Read the model definition and answer for the solid it produces. Units are mm, in the model's axes. A direction names the side the tool comes from. Round coordinates to 2 decimals unless told otherwise and drop trailing zeros. Order: outer loops, then holes, each group sorted by start corner. A loop starts at its lowest first (then second) coordinate and runs counter-clockwise, first axis right, second up. Notation, with made-up numbers: (22, 19.5) - (40, 19.5) arc R21 cw to (40, 25.5) - close; hole circle Ø5 at (47.25, -19.5). An arc over 180 degrees is marked (long way). One line per question, with ' | ' between items. Start each with the question number.
1) The part is cut by section B-B, the plane y = -30. Give the vertices of the cut face in (x, z).
2) The part is cut by section A-A, the plane x = 0. Give the vertices of the cut face in (y, z).
3) Straight lines are drawn through the part: line 1 (X direction, y = -8.7, z = 6); line 2 (X direction, y = -11.5, z = 6); line 3 (X direction, y = -13, z = 8.5). For each, find the intervals that lie inside material, in ascending order. Write a range as from..to.
4) The part is cut by section D-D, the plane x = 18. Give the vertices of the cut face in (y, z).
5) The part is cut by section C-C, the plane z = 6. Give the vertices of the cut face in (x, y).
6) The mould has two halves that part along Y. Classify faces 1 (the cylindrical face through (-51.29, -43.49, 6.08)), 2 (the flat face through (-31.4, 9.9, 12)), 3 (the cylindrical face through (-44.241, 25.877, 5.916)): pulls with the +Y half, pulls with the -Y half, needs draft (parallel to the pull), parting line crosses it, or undercut.
7) For faces 4 (the cylindrical face through (-37.69, 6.837, 5.916)), 5 (the flat face through (-52, -39, 6)), determine the directions among +Z, -Z, +X, -X, +Y, -Y from which every point of the face is accessible in a straight line to the end or side of a thin tool.
8) Flat-ended cylindrical pins translate along their axes: pin 1 (3.5 mm diameter, centred on x = -35.29, z = 6, fed in from -Y); pin 2 (2 mm diameter, centred on x = -14.5, z = 10, fed in from -Y); pin 3 (5 mm diameter, centred on x = -35.29, z = 6, fed in from +Y); pin 4 (4 mm diameter, centred on y = 22, z = 8.5, fed in from +X). Find the tip coordinate at first contact, or state that the pin passes through.
from build123d import *

# Parameters (mm, degrees)
F1_DEPTH = 12
F3_R     = 4
F3_R_2   = 2
F6_DEPTH = 100
F7_R     = 1


with BuildPart() as f1:
    # F0 (on Top) → F1 (new body)
    with BuildSketch(Plane.XY):
        with BuildLine():
            ThreePointArc((-30.9533166858, 9.9066738185), (32.5, 0), (-30.9533166858, -9.9066738185))
            ThreePointArc((-30.9533166858, -9.9066738185), (-36.1521865846, -6.4498953062), (-40.6700074334, -10.7588233268))
            ThreePointArc((-40.6700074334, -10.7588233268), (-44.1719937167, -25.6732051584), (-50.4508620887, -39.647413734))
            Line((-50.4508620887, -39.647413734), (-52, -35))
            Line((-52, -35), (-52, -45.9262987944))
            ThreePointArc((-52, -45.9262987944), (-43.3754164337, -29.3581013392), (-38.7212103105, -11.2686852631))
            ThreePointArc((-38.7212103105, -11.2686852631), (-38.6982701791, -11.0262325635), (-38.6558059993, -10.7864277375))
            ThreePointArc((-38.6558059993, -10.7864277375), (-35.9754973818, -8.4318261948), (-32.9297903997, -10.2897475302))
            ThreePointArc((-32.9297903997, -10.2897475302), (-32.8484099779, -10.5132023948), (-32.7849231086, -10.7423841283))
            ThreePointArc((-32.7849231086, -10.7423841283), (34.5, 0), (-32.7849231086, 10.7423841283))
            ThreePointArc((-32.7849231086, 10.7423841283), (-32.8484099779, 10.5132023948), (-32.9297903997, 10.2897475302))
            ThreePointArc((-32.9297903997, 10.2897475302), (-35.9754973818, 8.4318261948), (-38.6558059993, 10.7864277375))
            ThreePointArc((-38.6558059993, 10.7864277375), (-38.6982701791, 11.0262325635), (-38.7212103105, 11.2686852631))
            ThreePointArc((-38.7212103105, 11.2686852631), (-43.3754164337, 29.3581013392), (-52, 45.9262987944))
            Line((-52, 45.9262987944), (-52, 35))
            Line((-52, 35), (-50.4508620887, 39.647413734))
            ThreePointArc((-50.4508620887, 39.647413734), (-44.1719937167, 25.6732051584), (-40.6700074334, 10.7588233268))
            ThreePointArc((-40.6700074334, 10.7588233268), (-36.1521865846, 6.4498953062), (-30.9533166858, 9.9066738185))
        make_face()
        with BuildLine():
            ThreePointArc((-38.6558059993, -10.7864277375), (-38.6982701791, -11.0262325635), (-38.7212103105, -11.2686852631))
            ThreePointArc((-38.7212103105, -11.2686852631), (-38.6881506227, -11.0276049892), (-38.6558059993, -10.7864277375))
        make_face()
        with BuildLine():
            ThreePointArc((-38.6558059993, 10.7864277375), (-38.6881506227, 11.0276049892), (-38.7212103105, 11.2686852631))
            ThreePointArc((-38.7212103105, 11.2686852631), (-38.6982701791, 11.0262325635), (-38.6558059993, 10.7864277375))
        make_face()
        with BuildLine():
            ThreePointArc((-32.7849231086, -10.7423841283), (-32.8484099779, -10.5132023948), (-32.9297903997, -10.2897475302))
            ThreePointArc((-32.9297903997, -10.2897475302), (-32.8581361742, -10.5163152843), (-32.7849231086, -10.7423841283))
        make_face()
        with BuildLine():
            ThreePointArc((-32.7849231086, 10.7423841283), (-32.8581361742, 10.5163152843), (-32.9297903997, 10.2897475302))
            ThreePointArc((-32.9297903997, 10.2897475302), (-32.8484099779, 10.5132023948), (-32.7849231086, 10.7423841283))
        make_face()
    extrude(amount=F1_DEPTH)

    # F3 (on offset) → F4 (join, up to the next surface of F1)
    with BuildSketch(Plane.XZ.offset(15)):
        with Locations((-35.2927981995, 6)):
            Circle(F3_R)
        with Locations((-35.2927981995, 6)):
            Circle(F3_R_2, mode=Mode.SUBTRACT)
    extrude(until=Until.NEXT, dir=(0, 1, 0))

    # F5: F1 across plane


with BuildPart() as f1_1:
    add(f1.part)
    add(f1.part.mirror(Plane.XZ))

    # F3 (on offset) → F6 (cut)
    with BuildSketch(Plane.XZ.offset(15)):
        with Locations((-35.2927981995, 6)):
            Circle(F3_R_2)
    extrude(amount=-F6_DEPTH, mode=Mode.SUBTRACT)

    # F7
    f7_edges = [f1_1.edges().sort_by_distance(p)[0] for p in [
        (-52, -45.926299, 6),
        (-52, 45.926299, 6),
    ]]
    fillet(f7_edges, radius=F7_R)


solid = f1_1.part
Values:
1) outline: (-45.78, 0) - (-43.62, 0) - (-43.62, 12) - (-45.78, 12) - close; (-17.04, 0) - (-12.5, 0) - (-12.5, 12) - (-17.04, 12) - close; (12.5, 0) - (17.04, 0) - (17.04, 12) - (12.5, 12) - close
2) outline: (-34.5, 0) - (-32.5, 0) - (-32.5, 12) - (-34.5, 12) - close; (32.5, 0) - (34.5, 0) - (34.5, 12) - (32.5, 12) - close
3) line 1: x = -39.9..-37.29, -33.29..-31.53, 31.31..33.39 | line 2: x = -40.77..-37.29, -33.29..-30.4, 30.4..32.53 | line 3: x = -41.01..-38.98, -38.42..-32.17, -31.96..-29.79, 29.79..31.96
4) outline: (-29.43, 0) - (-27.06, 0) - (-27.06, 12) - (-29.43, 12) - close; (27.06, 0) - (29.43, 0) - (29.43, 12) - (27.06, 12) - close
5) outline: (-52, -42.53) arc R1 ccw to (-50.15, -43.06) arc R82.06 ccw to (-39.29, -14.82) - (-39.29, -15) - (-37.29, -15) - (-37.29, -6.69) arc R5 ccw to (-40.67, -10.76) arc R80.06 cw to (-50.45, -39.65) - (-52, -35) - close; (-52, 35) - (-50.45, 39.65) arc R80.06 cw to (-40.67, 10.76) arc R5 ccw to (-37.29, 6.69) - (-37.29, 15) - (-39.29, 15) - (-39.29, 14.82) arc R82.06 ccw to (-50.15, 43.06) arc R1 ccw to (-52, 42.53) - close; (-33.29, -15) - (-31.29, -15) - (-31.29, -14.53) arc R34.5 ccw (long way) to (-31.29, 14.53) - (-31.29, 15) - (-33.29, 15) - (-33.29, 7.06) arc R5 ccw to (-30.95, 9.91) arc R32.5 cw (long way) to (-30.95, -9.91) arc R5 ccw to (-33.29, -7.06) - close
6) face 1: pulls with the -Y half | face 2: needs draft | face 3: undercut
7) face 4: +Z, -Z | face 5: +Z, -Z, -X, +Y, -Y
8) pin 1: passes through | pin 2: stops at y = -31.75 | pin 3: stops at y = 15 | pin 4: stops at x = 28.11
